from build123d import *

# Parameters (mm, degrees)
EXTRUDE_1_DEPTH = 3
SKETCH_2_R      = 4
EXTRUDE_2_DEPTH = 43
CHAMFER_1_SIZE  = 0.1


with BuildPart() as part:
    # 草图1 → 凸台-拉伸1 (new body)
    with BuildSketch(Plane(origin=(0, 0, 0), x_dir=(1, 0, 0), z_dir=(0, 1, 0))):
        Polygon((0, 7.505553499), (-6.5, 3.75277675), (-6.5, -3.75277675), (0, -7.505553499), (6.5, -3.75277675), (6.5, 3.75277675), align=None)
    extrude(amount=EXTRUDE_1_DEPTH)

    # 草图2 → 凸台-拉伸2 (add)
    with BuildSketch(Plane.XZ):
        Circle(SKETCH_2_R)
    extrude(amount=EXTRUDE_2_DEPTH)

    # 倒角1
    chamfer_1_edges = [part.edges().sort_by_distance(p)[0] for p in [
        (-4, -43, 0),
    ]]
    chamfer(chamfer_1_edges, length=CHAMFER_1_SIZE)

    # 草图5 → 切除-旋转2 (revolve, cut)
    with BuildSketch(Plane(origin=(0, 0, 0), x_dir=(0, 0, -1), z_dir=(1, 0, 0))):
        Polygon((-6.945553499, 3), (-7.505553499, 2.44), (-7.505553499, 3), align=None)
        Polygon((-7.505553499, 0), (-7.505553499, 0.56), (-6.945553499, 0), align=None)
    revolve(axis=Axis((0, 3, 0), (0, 1, 0)), mode=Mode.SUBTRACT)


solid = part.part
Input: part model. Units: mm. Frame: model coordinates. A direction names the side the tool comes from. Coordinates: 2 decimals unless noted, no trailing zeros. Loops run counter-clockwise (first coordinate to the right, second up) from the corner with the lowest first, then second, coordinate; pieces in that order, holes last.
Q1. Material intervals for line 1 (Y direction, x = 2, z = -4.5); line 2 (Z direction, x = 0, y = -1); line 3 (X direction, y = -29, z = 0.5), sorted ascending.
Q2. Cut plane C-C (x = 4.75). Output: boundary loops of the cut face in (y, z).
Q3. Cut plane D-D (z = 6). Output: boundary loops of the cut face in (x, y).
Q4. Cut plane B-B (y = -14). Output: boundary loops of the cut face in (x, z).
Q5. Set-up query: faces 1 (the face through (-0.867, -21.15, -3.905)), 2 (the face through (-3.3, 1.5, 5.6)). Return all of +Z, -Z, +X, -X, +Y, -Y with unobstructed straight access to the full face (end or side cutting, diameter ignored); none if empty.
Q6. Cut plane A-A (z = 0). Output: boundary loops of the cut face in (x, y), then the cut area to 3 significant figures.
Q7. Contact query for flat-ended pins moving along their axis: pin 1 (3 mm diameter, centred on x = -2.5, y = -3, fed in from +Z); pin 2 (1.5 mm diameter, centred on y = -20, z = 3, fed in from -X); pin 3 (1 mm diameter, centred on y = -28.5, z = 3, fed in from +X). Output: stop coordinate, or through.
Working result:
1. line 1: y = 0 to 3
1. line 2: z = -4 to 4
1. line 3: x = -3.97 to 3.97
2. outline: (0, -4.76) - (3, -4.76) - (3, 4.76) - (0, 4.76) - close
3. outline: (-2.61, 0) - (2.61, 0) - (2.61, 3) - (-2.61, 3) - close
4. outline: circle Ø8 at (0, 0)
5. face 1: -Y
5. face 2: +Z, -X, +Y, -Y
6. outline: (-6.5, 0) - (-4, 0) - (-4, -42.9) - (-3.9, -43) - (3.9, -43) - (4, -42.9) - (4, 0) - (6.5, 0) - (6.5, 3) - (-6.5, 3) - close
6. area: 383 mm2
7. pin 1: stops at z = 3.87
7. pin 2: stops at x = -3.31
7. pin 3: stops at x = 3.12
